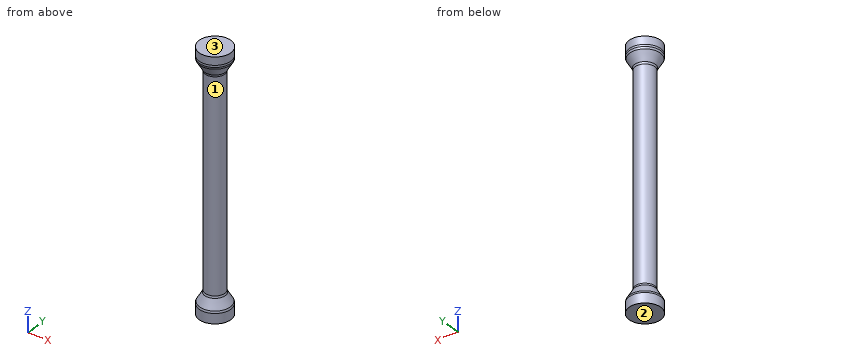
from build123d import *

# Parameters (mm, degrees)
F0_W        = 4.9
F0_H        = 60
F2_S5_R     = 8
F2_T6_DEPTH = 15
F3_S5_R     = 8
F3_T6_DEPTH = 15
F4_R        = 2


# Not quite as in the source:
# - a fillet or chamfer that OpenCascade refuses, or shapes differently, is made with other operations: its cross-section is extruded or revolved along the edge and cut away or added


with BuildPart() as f1:
    # F0 (on Front) → F1 (revolve)
    with BuildSketch(Plane.XZ):
        Polygon((0, 64), (0, 60), (4.9, 60), (8, 60), (8, 64), align=None)
        with Locations((2.45, 30)):
            Rectangle(F0_W, F0_H)
        with Locations((2.45, -30)):
            Rectangle(F0_W, F0_H)
        Polygon((4.9, -60), (0, -60), (0, -64), (8, -64), (8, -60), align=None)
    revolve(axis=Axis((0, 0, -30), (0, 0, -1)))

    # F2: chamfer of 4 x 6.9282032303 on 1 edges, made by hand


with BuildPart() as f2_tool2:
    # F2_s3 → F2_t4 (revolve)
    with BuildSketch(Plane.XZ):
        Polygon((4.9, 53.0717967697), (8.9, 60), (4.9, 60), align=None)
    revolve(axis=Axis((0, 0, 60), (0, 0, -1)))

    # F2_s5 → F2_t6 (intersect, symmetric)
    with BuildSketch(Plane.XY.offset(56.5)):
        Circle(F2_S5_R)
    extrude(amount=F2_T6_DEPTH, both=True, mode=Mode.INTERSECT)


with BuildPart() as f1_1:
    add(f1.part)

    # F2_t1: union F2_tool2
    add(f2_tool2.part)

    # F3: chamfer of 4 x 6.9282032303 on 1 edges, made by hand


with BuildPart() as f3_tool2:
    # F3_s3 → F3_t4 (revolve)
    with BuildSketch(Plane.XZ):
        Polygon((8.9, -60), (4.9, -53.0717967697), (4.9, -60), align=None)
    revolve(axis=Axis((0, 0, -60), (0, 0, -1)))

    # F3_s5 → F3_t6 (intersect, symmetric)
    with BuildSketch(Plane.XY.offset(-56.5)):
        Circle(F3_S5_R)
    extrude(amount=F3_T6_DEPTH, both=True, mode=Mode.INTERSECT)


with BuildPart() as f1_2:
    add(f1_1.part)

    # F3_t1: union F3_tool2
    add(f3_tool2.part)

    # F4
    f4_edges = [f1_2.edges().sort_by_distance(p)[0] for p in [
        (-8, 0, -58.441154),
        (-4.9, 0, -53.071797),
        (-4.9, 0, 53.071797),
        (-8, 0, 58.441154),
    ]]
    fillet(f4_edges, radius=F4_R)


solid = f1_2.part
Input: part model. Units: mm. Frame: model coordinates. Face numbers are marked on the shaded views. Give positions to 0.01 mm unless a question says otherwise; leave off trailing zeros. Order: outer loops, then holes, each group sorted by start corner. A loop starts at its lowest first (then second) coordinate and runs counter-clockwise, first axis right, second up.
Q1. Draft query along Z for the marked faces 1, 2 and 3. Return one class per face: +Z half, -Z half, draft (parallel to the pull), parting line (faces both ways), or undercut.
Checked values:
face 1: undercut
face 2: -Z half
face 3: +Z half
Q2. Contact query for flat-ended pins moving along their axis: pin 1 Ø4 at (y, z) = (1, -43.5) entering from +X; pin 2 Ø1.5 at (x, z) = (6, -5) entering from -Y; pin 3 Ø2 at (x, z) = (-5.5, 22.5) entering from -Y. Output: stop coordinate, or through.
Checked values:
pin 1: stops at x = 4.9
pin 2: passes through
pin 3: stops at y = -1.94
Q3. Section A-A on z = -36.5. Output: boundary loops of the cut face in (x, y), and give its area (3 significant figures).
Checked values:
outline: circle Ø9.8 at (0, 0)
area: 75.4 mm2
Q4. Section B-B on z = 55.5. Output: boundary loops of the cut face in (x, y), and give its area (3 significant figures).
Checked values:
outline: circle Ø12.6 at (0, 0)
area: 125 mm2
Q5. Ray query, probe 1 along X at (y, z) = (0.25, -10); probe 2 along Z at (x, y) = (5, 3.25); probe 3 along Y at (x, z) = (0, 33.5). Return the intervals inside material, ascending.
Checked values:
probe 1: x = -4.89 to 4.89
probe 2: z = -64 to -54.91, 54.91 to 64
probe 3: y = -4.9 to 4.9
